Autodesk Inventor part; units mm, degrees
ref_plane "YZ Plane" through (0, 0, 0) normal (1, 0, 0) x (0, 1, 0)
ref_plane "XZ Plane" through (0, 0, 0) normal (0, 1, 0) x (-1, 0, 0)
ref_plane "XY Plane" through (0, 0, 0) normal (0, 0, 1) x (1, 0, 0)
sketch "Sketch1" plane through (0, 0, 0) normal (0, 1, 0) x (-1, 0, 0)
  line L0 (0, 0) -> (152.4, 0)
  line L1 (152.4, 0) -> (152.4, 252.095)
  line L2 (152.4, 252.095) -> (0, 252.095)
  line L3 (0, 252.095) -> (0, 0)
  circle A0 centre (76.2, 76.2) radius 50.8
  circle A1 centre (76.2, 76.2) radius 4.5
  dimension "d0" = 152.4
  dimension "d1" = 252.095
  dimension "d2" = 101.6
  dimension "d3" = 9
extrude "Extrusion1" add sketch "Sketch1" against normal blind 3.175 contours L3 L2 L1 L0 | A0
sketch "Sketch2" plane through (0, 0, 0) normal (0, 1, 0) x (1, 0, 0)
  line L0 (0, -252.095) -> (-152.4, -252.095)
  line L1 (-152.4, -252.095) -> (-152.4, 0)
  line L2 (0, -252.095) -> (-152.4, -252.095)
  line L3 (-152.4, -252.095) -> (-152.4, -248.92)
  line L4 (-152.4, -248.92) -> (0, -248.92)
  line L5 (0, -248.92) -> (0, -252.095)
  point P0 (0, 0)
  dimension "d6" = 3.175
extrude "Extrusion2" add sketch "Sketch2" along normal blind 25.4
sketch "Sketch3" plane through (0, 0, 0) normal (0, 1, 0) x (1, 0, 0)
  circle A0 centre (-66.421, -76.2) radius 2
  circle A1 centre (-85.979, -76.2) radius 2
  circle A2 centre (-76.2, -66.421) radius 2
  circle A3 centre (-76.2, -85.979) radius 2
  point P0 (0, 0)
  dimension "d9" = 4
  dimension "d10" = 4
  dimension "d11" = 4
  dimension "d12" = 4
extrude "Extrusion3" cut sketch "Sketch3" against normal blind 25.4
sketch "Sketch4" plane through (0, 0, 0) normal (0, 1, 0) x (1, 0, 0)
  circle A0 centre (-76.2, -85.979) radius 2
  circle A1 centre (-76.2, -85.979) radius 2
  circle A2 centre (-76.2, -76.2) radius 4.5
  circle A3 centre (-76.2, -76.2) radius 4.5
  circle A4 centre (-83.1148, -83.1148) radius 2
  circle A5 centre (-76.2, -76.2) radius 4.5
  circle A6 centre (-85.979, -76.2) radius 2
  circle A7 centre (-76.2, -76.2) radius 4.5
  circle A8 centre (-83.1148, -69.2852) radius 2
  circle A9 centre (-76.2, -76.2) radius 4.5
  circle A10 centre (-76.2, -66.421) radius 2
  circle A11 centre (-76.2, -76.2) radius 4.5
  circle A12 centre (-69.2852, -69.2852) radius 2
  circle A13 centre (-76.2, -76.2) radius 4.5
  circle A14 centre (-66.421, -76.2) radius 2
  circle A15 centre (-76.2, -76.2) radius 4.5
  circle A16 centre (-69.2852, -83.1148) radius 2
  circle A17 centre (-76.2, -76.2) radius 4.5
  point P0 (0, 0)
  dimension "d17" = 360
extrude "Extrusion4" cut sketch "Sketch4" against normal blind 25.4 contours A4 | A8 | A12 | A16
sketch "Sketch5" plane through (0, 0, 0) normal (0, 1, 0) x (1, 0, 0)
  point P0 (0, 0)
sketch "Sketch6" plane through (0, 0, 0) normal (0, 1, 0) x (1, 0, 0)
  point P0 (0, 0)
sketch "Sketch7" plane through (0, -3.175, 0) normal (0, -1, 0) x (1, 0, 0)
  circle A0 centre (-83.1148, 83.1148) radius 2
  circle A1 centre (-83.1148, 83.1148) radius 2.8284
  circle A2 centre (-83.1148, 69.2852) radius 2
  circle A3 centre (-83.1148, 69.2852) radius 2.8284
  circle A4 centre (-69.2852, 69.2852) radius 2
  circle A5 centre (-69.2852, 69.2852) radius 2.9799
  circle A6 centre (-69.2852, 83.1148) radius 29.4992
  circle A7 centre (-69.2852, 83.1148) radius 2
  circle A8 centre (-69.2852, 83.1148) radius 3.4641
  point P0 (0, 0)
extrude "Extrusion5" add sketch "Sketch7" against normal blind 3.175 contours A0 | A1 | A2 | A3 | A4 | A5 | A7 | A8
sketch "Sketch8" plane through (0, 0, 0) normal (0, 1, 0) x (1, 0, 0)
  circle A0 centre (-76.2, -76.2) radius 4.5
  circle A1 centre (-76.2, -76.2) radius 4.5
  circle A2 centre (-64.2, -76.2) radius 2
  circle A3 centre (-76.2, -76.2) radius 4.5
  circle A4 centre (-76.2, -76.2) radius 4.5
  circle A5 centre (-76.2, -76.2) radius 4.5
  circle A6 centre (-76.2, -76.2) radius 4.5
  circle A7 centre (-76.2, -76.2) radius 4.5
  circle A8 centre (-76.2, -76.2) radius 4.5
  circle A9 centre (-76.2, -76.2) radius 4.5
  circle A10 centre (-67.7147, -84.6853) radius 2
  circle A11 centre (-84.6853, -84.6853) radius 2
  circle A12 centre (-84.6853, -67.7147) radius 2
  circle A13 centre (-67.7147, -67.7147) radius 2
  point P0 (0, 0)
  point P1 (-76.2, -64.2)
  point P2 (-88.2, -76.2)
  point P3 (-76.2, -88.2)
  dimension "d23" = 4
  dimension "d26" = 360
  dimension "d28" = 4
  dimension "d29" = 4
  dimension "d30" = 4
  dimension "d31" = 4
extrude "Extrusion6" cut sketch "Sketch8" against normal blind 25.4 contours A10 | A11 | A12 | A13
sketch "Sketch9" plane through (0, 25.4, 0) normal (0, 1, 0) x (1, 0, 0)
  line L0 (0, -248.92) -> (0, 0)
  line L1 (-163.9684, -278.6073) -> (0, -278.6073)
  line L2 (0, -278.6073) -> (0, -205.6552)
  line L3 (0, -205.6552) -> (-163.9684, -205.6552)
  line L4 (-163.9684, -205.6552) -> (-163.9684, -278.6073)
extrude "Extrusion7" cut sketch "Sketch9" against normal blind 25.4
sketch "Sketch10" plane through (0, 0, 0) normal (0, 1, 0) x (1, 0, 0)
  line L0 (-152.4, -252.095) -> (-152.4, 0)
  line L1 (0, -101.6) -> (-152.4, -101.6)
  line L2 (-152.4, -101.6) -> (-152.4, -252.095)
  line L3 (-152.4, -252.095) -> (0, -252.095)
  line L4 (0, -252.095) -> (0, -101.6)
  point P0 (0, 0)
extrude "Extrusion8" add sketch "Sketch10" along normal blind 18.288
sketch "Sketch11" plane through (0, 18.288, 0) normal (0, 1, 0) x (1, 0, 0)
  point P0 (0, 0)
sketch "Sketch12" plane through (0, 18.288, 0) normal (0, 1, 0) x (1, 0, 0)
  line L0 (0, -252.095) -> (-152.4, -252.095)
  line L1 (-152.4, -252.095) -> (0, -252.095)
  line L2 (0, -252.095) -> (0, -248.92)
  line L3 (0, -248.92) -> (-152.4, -248.92)
  line L4 (-152.4, -248.92) -> (-152.4, -252.095)
  point P0 (0, 0)
  dimension "d38" = 3.175
extrude "Extrusion9" add sketch "Sketch12" along normal blind 25.4
sketch "Sketch13" plane through (0, -3.175, 252.095) normal (1, 0, 0) x (0, 0, -1)
  line L0 (150.495, 3.175) -> (150.495, 21.463)
  line L1 (0, 0) -> (0, 46.863)
  line L2 (150.495, 21.463) -> (0, 21.463)
  line L3 (0, 21.463) -> (0, 18.288)
  line L4 (0, 18.288) -> (150.495, 18.288)
  line L5 (150.495, 18.288) -> (150.495, 21.463)
  line L6 (252.095, 0) -> (0, 0)
  line L7 (150.495, 21.463) -> (147.32, 21.463)
  line L8 (147.32, 21.463) -> (147.32, 0)
  line L9 (147.32, 0) -> (150.495, 0)
  line L10 (150.495, 0) -> (150.495, 21.463)
  line L11 (0, 18.288) -> (147.32, 18.288)
  line L12 (147.32, 18.288) -> (147.32, 0)
  line L13 (147.32, 0) -> (0, 0)
  line L14 (0, 0) -> (0, 18.288)
  point P0 (252.095, 3.175)
  dimension "d41" = 3.175
  dimension "d42" = 3.175
extrude "Extrusion10" cut sketch "Sketch13" against normal blind 254 contours L8 L6 L1 L4
properties part number "Single Sided board"
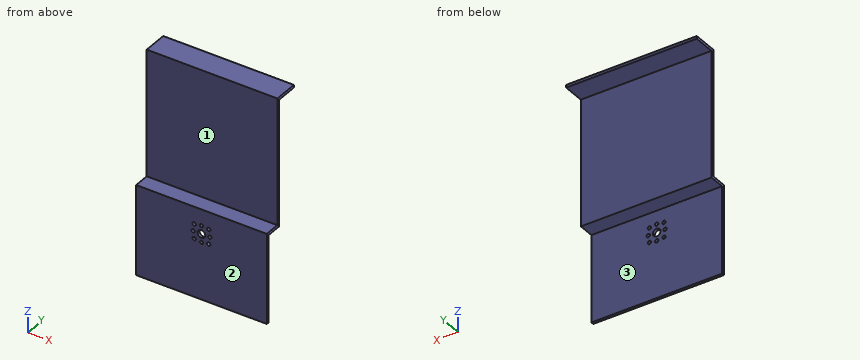
Read the model definition and answer for the solid it produces. Units are mm, in the model's axes. Face numbers are marked on the shaded views. A direction names the side the tool comes from. Coordinates: 2 decimals unless noted, no trailing zeros. Loops run counter-clockwise (first coordinate to the right, second up) from the corner with the lowest first, then second, coordinate; pieces in that order, holes last. Notation, with made-up numbers: (-18.75, 68) -> (-3.75, 68) arc R31 cw to (-3.75, 102) -> close; hole circle Ø1 at (43, -29.5). An arc over 180 degrees is marked (long way). Answer in a Markdown table with one row per item.
Item 1: Each of these flat-tipped pins is pushed along its axis until it touches: P1, Ø12, axis at x = -45.5, z = 165, coming from the -Y side; P2, Ø9, axis at x = -65, y = 4.5, coming from the +Z side (3 decimals); P3, Ø5.5, axis at x = -67, y = 6, coming from the -Z side. Where does it stop, or does it pass through?
Returned:
| item | result |
|---|---|
| P1 | stops at y = 15.11 |
| P2 | stops at z = 104.775 |
| P3 | stops at z = 101.6 |
Item 2: For the marked faces 1, 2 and 3, determine the directions among +Z, -Z, +X, -X, +Y, -Y from which every point of the face is accessible in a straight line to the end or side of a thin tool.
Returned:
| item | result |
|---|---|
| face 1 | +Z, +X, -X, -Y |
| face 2 | +Z, -Z, +X, -X, -Y |
| face 3 | -Z, +X, -X, +Y |
Item 3: A cutting plane is placed at C-C on y = 12. Determine the outline of the cut face in (x, z) (3 decimals), plus the area to 3 significant figures.
Returned:
| item | result |
|---|---|
| outline | (-152.4, 101.6) -> (0, 101.6) -> (0, 104.775) -> (-152.4, 104.775) -> close |
| area | 484 mm^2 |
Item 4: A cutting plane is placed at A-A on x = -17. Determine the outline of the cut face in (y, z) (3 decimals).
Returned:
| item | result |
|---|---|
| outline | (-3.175, 0) -> (0, 0) -> (0, 101.6) -> (18.288, 101.6) -> (18.288, 248.92) -> (43.688, 248.92) -> (43.688, 252.095) -> (15.113, 252.095) -> (15.113, 104.775) -> (-3.175, 104.775) -> close |
Item 5: A cutting plane is placed at B-B on z = 173. Determine the outline of the cut face in (x, y).
Returned:
| item | result |
|---|---|
| outline | (-152.4, 15.11) -> (0, 15.11) -> (0, 18.29) -> (-152.4, 18.29) -> close |
Item 6: Straight lines are drawn through the part: line 1 along Z through (x, y) = (-76.2, -0.9) (3 decimals); line 2 along X through (y, z) = (-1, 76); line 3 along Z through (x, y) = (-95, 13) (3 decimals). For each, find the intervals that lie inside material, in ascending order. Write a range as [from, to].
Returned:
| item | result |
|---|---|
| line 1 | z = [0, 64.421], [68.421, 71.7], [80.7, 83.979], [87.979, 104.775] |
| line 2 | x = [-152.4, -87.97], [-83.99, -80.7], [-71.7, -68.41], [-64.43, 0] |
| line 3 | z = [101.6, 104.775] |
